Check sheet for the modelled part. Datum: model origin and axes. Units: mm. Face numbers are marked on the shaded views. Give positions to 0.01 mm unless a question says otherwise; leave off trailing zeros. Order: outer loops, then holes, each group sorted by start corner. A loop starts at its lowest first (then second) coordinate and runs counter-clockwise, first axis right, second up. Notation, with made-up numbers: (25.25, -7) -> (44.25, -7) arc R20 cw to (44.25, 7) -> close; hole circle Ø10 at (24, -31.5). An arc over 180 degrees is marked (long way). Answer in a Markdown table with one row per item. Add a question column.
(1) Thickness scan on L1, parallel to Y at x = 30, z = -13.25; L2, parallel to Y at x = 21, z = -8.5; L3, parallel to X at y = -173, z = -12.75 (3 decimals). Record the ranges inside material, lowest first. Write a range as [from, to].
(2) Cross-section at A-A (z = -13.25). Record the cut outline in (x, y) (1 decimal), then the cut area to 3 significant figures.
(3) Cross-section at D-D (x = 22.5). State how many separate pieces and enclosed holes the cut face has, then the cut area to 3 significant figures.
(4) Cross-section at C-C (y = -141). Record the cut outline in (x, z) (3 decimals), then the cut area to 3 significant figures.
(5) Cross-section at B-B (x = 7). Record the cut outline in (y, z) (3 decimals), then the cut area to 3 significant figures.
(6) Go/stop test with flat-tipped pins: pin 1 (5 mm diameter, centred on x = 32.5, y = -158, fed in from +Z); pin 2 (11.5 mm diameter, centred on x = 23.81, y = -161.93, fed in from -Z); pin 3 (3.5 mm diameter, centred on y = -125, z = -13, fed in from -X) (3 decimals); pin 4 (4.5 mm diameter, centred on x = 4, y = -54, fed in from -Z). Record where each tip stops, or that it passes through.
(7) Release check for a two-part mould opening along Y. For the marked faces 1, 2 and 3 record: released by +Y, released by -Y, zero draft, split by the parting line, or undercut.
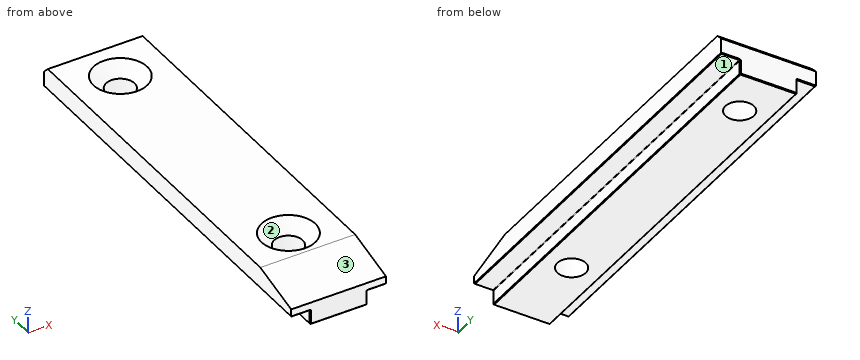
```python
from build123d import *

# Parameters (mm, degrees)
F1_DEPTH       = 203.2
F3_DEPTH       = 47.626
F5_D           = 14.2748
F5_CSINK_D     = 26.9748
F5_CSINK_ANGLE = 90
F6_SIZE        = 3.175
F7_R           = 0.254
F8_SIZE        = 0.381


with BuildPart() as f1:
    # F0 (on Front) → F1 (new body)
    with BuildSketch(Plane.XZ):
        Polygon((47.625, 0), (0, 0), (0, -10.8712), (9.525, -10.8712), (9.525, -18.2372), (38.1, -18.2372), (38.1, -10.8712), (47.625, -10.8712), align=None)
    extrude(amount=F1_DEPTH)

    # F2 (on face) → F3 (cut, through all)
    with BuildSketch(Plane(origin=(0, 0, 0), x_dir=(0, -1, 0), z_dir=(-1, 0, 0))):
        Polygon((203.2, -6.805909), (203.2, 0), (177.8, 0), align=None)
    extrude(amount=-F3_DEPTH, mode=Mode.SUBTRACT)

    # F5 (through all)
    with Locations(Plane.XY):
        with Locations((23.8125, -23.8125), (23.8125, -161.925)):
            CounterSinkHole(F5_D / 2, F5_CSINK_D / 2, counter_sink_angle=F5_CSINK_ANGLE)

    # F6
    f6_edges = [f1.edges().sort_by_distance(p)[0] for p in [
        (23.8125, 0, 0),
    ]]
    chamfer(f6_edges, length=F6_SIZE)

    # F7
    f7_edges = [f1.edges().sort_by_distance(p)[0] for p in [
        (9.525, -101.6, -10.8712),
        (38.1, -101.6, -10.8712),
    ]]
    fillet(f7_edges, radius=F7_R)

    # F8
    f8_edges = [f1.edges().sort_by_distance(p)[0] for p in [
        (38.1, -101.6, -18.2372),
        (9.525, -101.6, -18.2372),
        (23.8125, -203.2, -18.2372),
        (23.8125, 0, -18.2372),
        (38.1, 0, -14.6812),
        (9.525, 0, -14.6812),
        (9.525, -203.2, -14.6812),
        (38.1, -203.2, -14.6812),
        (47.625, -101.6, -10.8712),
        (0, -101.6, -10.8712),
    ]]
    chamfer(f8_edges, length=F8_SIZE)


solid = f1.part
```
Answer below:
| question | item | result |
|---|---|---|
| 1 | L1 | y = [-203.2, -165.48], [-158.37, -27.37], [-20.25, 0] |
| 1 | L2 | y = [-203.2, -168.48], [-155.37, -30.37], [-17.25, 0] |
| 1 | L3 | x = [9.525, 38.1] |
| 2 | outline | (9.5, -202.8) -> (9.9, -203.2) -> (37.7, -203.2) -> (38.1, -202.8) -> (38.1, -0.4) -> (37.7, 0) -> (9.9, 0) -> (9.5, -0.4) -> close; hole circle Ø14.3 at (23.8, -161.9); hole circle Ø14.3 at (23.8, -23.8) |
| 2 | area | 5,490 mm² |
| 3 | separate pieces | 3 |
| 3 | enclosed holes | 0 |
| 3 | area | 3,020 mm² |
| 4 | outline | (0, -10.49) -> (0.381, -10.871) -> (9.271, -10.871) arc R0.254 cw to (9.525, -11.125) -> (9.525, -17.856) -> (9.906, -18.237) -> (37.719, -18.237) -> (38.1, -17.856) -> (38.1, -11.125) arc R0.254 cw to (38.354, -10.871) -> (47.244, -10.871) -> (47.625, -10.49) -> (47.625, 0) -> (0, 0) -> close |
| 4 | area | 728 mm² |
| 5 | outline | (-203.2, -10.49) -> (-202.819, -10.871) -> (-0.381, -10.871) -> (0, -10.49) -> (0, -3.175) -> (-3.175, 0) -> (-177.8, 0) -> (-203.2, -6.806) -> close |
| 5 | area | 2,120 mm² |
| 6 | pin 1 | stops at z = -1.45 |
| 6 | pin 2 | passes through |
| 6 | pin 3 | stops at x = 9.525 |
| 6 | pin 4 | stops at z = -10.87 |
| 7 | face 1 | zero draft |
| 7 | face 2 | undercut |
| 7 | face 3 | released by -Y |
